from build123d import *

# Parameters (mm, degrees)
F1_DEPTH = 3.175
F0_W     = 3.175
F0_H     = 101.9676364958
F2_DEPTH = 76.2
F4_DEPTH = 106.68


with BuildPart() as f1:
    # F0 (on Top) → F1 (new body)
    with BuildSketch(Plane.XY):
        Polygon((25.4167113453, 75.9493410587), (0, 75.9493410587), (-25.4167113453, 75.9493410587), (-38.3506603539, 50.683028996), (-38.3506603539, -51.2846074998), (-25.4167113453, -76.5509232879), (0, -76.5509232879), (25.4167113453, -76.5509232879), (38.3506603539, -51.2846074998), (38.3506603539, 50.683028996), align=None)
    extrude(amount=F1_DEPTH)

    # F0 (on Top) → F2 (join)
    with BuildSketch(Plane.XY):
        Polygon((-25.4167113453, 75.9493410587), (0, 75.9493410587), (25.4167113453, 75.9493410587), (25.4167113453, 79.1243410587), (-25.4167113453, 79.1243410587), align=None)
        Polygon((-38.3506603539, 50.683028996), (-25.4167113453, 75.9493410587), (-28.5917113453, 75.9493410587), (-41.5256603539, 50.683028996), (-41.5256603539, -51.2846074998), (-28.5917113453, -76.5509232879), (-27.9901291162, -76.5509232879), (-25.4167113453, -76.5509232879), (-38.3506603539, -51.2846074998), align=None)
        Polygon((-28.5917113453, 75.9493410587), (-25.4167113453, 75.9493410587), (-25.4167113453, 79.1243410587), align=None)
        Polygon((28.5917113453, 75.9493410587), (25.4167113453, 75.9493410587), (38.3506603539, 50.683028996), (41.5256603539, 50.683028996), align=None)
        Polygon((25.4167113453, 79.1243410587), (25.4167113453, 75.9493410587), (28.5917113453, 75.9493410587), align=None)
        with Locations((39.9381603539, -0.3007892519)):
            Rectangle(F0_W, F0_H)
        Polygon((41.5256603539, -51.2846074998), (38.3506603539, -51.2846074998), (25.4167113453, -76.5509232879), (27.9901291162, -76.5509232879), (28.5917113453, -76.5509232879), align=None)
        Polygon((-25.4167113453, -79.1243410587), (-25.4167113453, -76.5509232879), (-27.9901291162, -76.5509232879), align=None)
        Polygon((0, -76.5509232879), (-25.4167113453, -76.5509232879), (-25.4167113453, -79.1243410587), (25.4167113453, -79.1243410587), (25.4167113453, -76.5509232879), align=None)
        Polygon((27.9901291162, -76.5509232879), (25.4167113453, -76.5509232879), (25.4167113453, -79.1243410587), align=None)
    extrude(amount=F2_DEPTH)

    # F3 (on face) → F4 (cut)
    with BuildSketch(Plane.YZ.offset(41.5256603539)):
        with BuildLine():
            ThreePointArc((5.5000017, 38.1), (-3.8890884986, 41.9890884986), (0, 32.5999983))
            ThreePointArc((0, 32.5999983), (3.8890884986, 34.2109115014), (5.5000017, 38.1))
        make_face()
    extrude(amount=-F4_DEPTH, mode=Mode.SUBTRACT)


solid = f1.part
Design review of the part built by this model. Coordinates are the model's own, in mm. A direction names the side the tool comes from. Round coordinates to 2 decimals unless told otherwise and drop trailing zeros. Loops run counter-clockwise (first coordinate to the right, second up) from the corner with the lowest first, then second, coordinate; pieces in that order, holes last. Notation, with made-up numbers: (76, 79.25) - (89, 79.25) arc R13 ccw to (89, 99.25) - close; hole circle Ø11 at (41, 32.25). An arc over 180 degrees is marked (long way). One line per item, written item: value. Start each with the question number.
1) Consider section C-C on y = -31. Give the boundary of the cut face in (x, z) (3 decimals), then the cut area to 3 significant figures.
2) Draft analysis for pull direction X (two halves, no side actions). For faces 3 (the flat face through (-35.15, -63.74, 37.57)), 4 (the flat face through (-38.351, -1, 47)), 5 (the flat face through (-1, 1, 0)), 6 (the flat face through (27.03, 77.51, 37.57)), state which applies: +X half, -X half, draft (parallel to the pull), parting line (faces both ways), or undercut.
3) Consider section A-A on z = 13. Give the boundary of the cut face in (x, y).
4) Insertion check: pin 1 Ø0.5 at (x, z) = (28.5, 27) entering from -Y; pin 2 Ø14.5 at (y, z) = (0, 38.1) entering from -X; pin 3 Ø1.5 at (x, y) = (-0.5, 18.5) entering from +Z (3 decimals); pin 4 Ø3 at (x, z) = (27.5, 37) entering from -Y. Each pin has a flat end and moves straight along its axis. Give the tip position at first contact, or say it passes through.
5) For faces 1 (the flat face through (0, -79.124, 38)), 2 (the flat face through (0, -76.551, 39)), list the 3-axis set-ups (+Z, -Z, +X, -X, +Y, -Y) from which the entire face can be reached by the end or side of a thin tool; tool diameter is ignored.
6) To check wall thickness, follow L1, parallel to X at y = 36, z = 43; L2, parallel to Y at x = -4, z = 20.5; L3, parallel to Y at x = -36, z = 5. State the ranges of each line that lie inside material, in increasing order. Write a range as from..to.
7) Consider section B-B on x = 16.5. Give the boundary of the cut face in (y, z) (3 decimals).
Reported:
1. outline: (-41.526, 0) - (41.526, 0) - (41.526, 76.2) - (38.351, 76.2) - (38.351, 3.175) - (-38.351, 3.175) - (-38.351, 76.2) - (-41.526, 76.2) - close
1. area: 727 mm^2
2. face 3: -X half
2. face 4: undercut
2. face 5: draft
2. face 6: +X half
3. outline: (-41.53, -51.28) - (-28.59, -76.55) - (-27.99, -76.55) - (-25.42, -79.12) - (25.42, -79.12) - (27.99, -76.55) - (28.59, -76.55) - (41.53, -51.28) - (41.53, 50.68) - (28.59, 75.95) - (25.42, 79.12) - (-25.42, 79.12) - (-28.59, 75.95) - (-41.53, 50.68) - close; hole (-38.35, -51.28) - (-25.42, -76.55) - (25.42, -76.55) - (38.35, -51.28) - (38.35, 50.68) - (25.42, 75.95) - (-25.42, 75.95) - (-38.35, 50.68) - close
4. pin 1: stops at y = -76.55
4. pin 2: stops at x = -41.53
4. pin 3: stops at z = 3.175
4. pin 4: stops at y = -78.54
5. face 1: +Z, -Z, +X, -X, -Y
5. face 2: +Z
6. L1: x = -41.53..-38.35, 38.35..41.53
6. L2: y = -79.12..-76.55, 75.95..79.12
6. L3: y = -62.08..-55.88, 55.28..61.48
7. outline: (-79.124, 0) - (79.124, 0) - (79.124, 76.2) - (75.949, 76.2) - (75.949, 3.175) - (-76.551, 3.175) - (-76.551, 76.2) - (-79.124, 76.2) - close
